Source: CAD feature listing. Evaluate the final solid. Frame: model axes, mm. A direction names the side the tool comes from. Coordinates: 2 decimals unless noted, no trailing zeros. Write each loop counter-clockwise with the first axis right and the second up, starting at its lowest first coordinate (ties: lowest second). Pieces come first, ordered by that corner, then holes. Notation, with made-up numbers: M 0.25,77.5 L 16.25,77.5 A7 cw 16.25,84.5 Z; hole C 82.25,69 d1. An arc over 180 degrees is marked long. One line per item, written item: value. Start each with the question number.
Item 1: Ray query, L1, parallel to Z at x = 30.5, y = 0; L2, parallel to X at y = 1, z = 43; L3, parallel to X at y = -4.5, z = 7.5. Return the intervals inside material, ascending. Write a range as from..to.
Item 2: Cut plane A-A, the plane z = 57. Output: boundary loops of the cut face in (x, y).
Item 3: Mould query, pull axis X, two halves, no side actions, for faces 1 (the flat face through (1, 2, 74.953)), 2 (the conical face through (23.188, -7.238, 0.016)), 3 (the conical face through (19.34, 12.68, 7.42)). Classes: released by +X, released by -X, zero draft, split by the parting line, or undercut.
Item 4: Pin query (flat end, axial travel): P1, Ø5, axis at x = -13, y = -33.5, coming from the +Z side; P2, Ø4, axis at x = -34, y = -13, coming from the +Z side; P3, Ø1, axis at x = -16, y = 20.5, coming from the -Z side. Return the tip coordinate at first contact, or that it passes through.
Item 5: Set-up query: faces 4 (the conical face through (15.18, 9.84, 14.57)), 5 (the conical face through (-14.935, 9.014, 14.993)), 6 (the conical face through (-0.628, 2.83, -14.225)). Return all of +Z, -Z, +X, -X, +Y, -Y with unobstructed straight access to the full face (end or side cutting, diameter ignored); none if empty.
```python
from build123d import *

# Parameters (mm, degrees)
F3_DEPTH = 74.9529767781


with BuildPart() as f1:
    # F0 (on Front) → F1 (revolve)
    with BuildSketch(Plane.XZ):
        Polygon((0.4052141029, 14.5266056061), (0.2008356291, 0), (23.175150156, 0), (23.175150156, 14.5266056061), (11.587575078, 14.5266056061), align=None)
        Polygon((0.2008356291, 0), (0, -14.2747908831), (46.350300312, -14.2747908831), (46.350300312, 0), (23.175150156, 0), align=None)
        Polygon((0.9806752205, 55.4286465049), (0.4052141029, 14.5266056061), (11.587575078, 14.5266056061), (11.9791924953, 55.4286465049), align=None)
    revolve(axis=Axis((0.4903376102, 0, 20.5769278109), (-0.0140678597, 0, -0.9999010428)))

    # F2 (on Top) → F3 (join)
    with BuildSketch(Plane.XY):
        Polygon((-26.0949339381, -15.407031402), (28.0455284658, -15.407031402), (0, 27.8120934963), align=None)
    extrude(amount=F3_DEPTH)


solid = f1.part
```
From the geometry:
1. L1: z = -14.27..0
1. L2: x = -16.19..17.4
1. L3: x = -22.12..22.73
2. outline: M -26.09,-15.41 L 28.05,-15.41 L 0,27.81 Z
3. face 1: zero draft
3. face 2: undercut
3. face 3: released by +X
4. P1: stops at z = 0.75
4. P2: stops at z = 1.05
4. P3: stops at z = -13.7
5. face 4: +Z, +X
5. face 5: +Z
5. face 6: -Z, -X
